Could you check a few things on this drawing? It's one solid part, dimensions in mm from its lowest x, y, z. Give positions to 0.01 mm unless a question says otherwise; leave off trailing zeros. Answer as a JSON object with one key per item and string values.
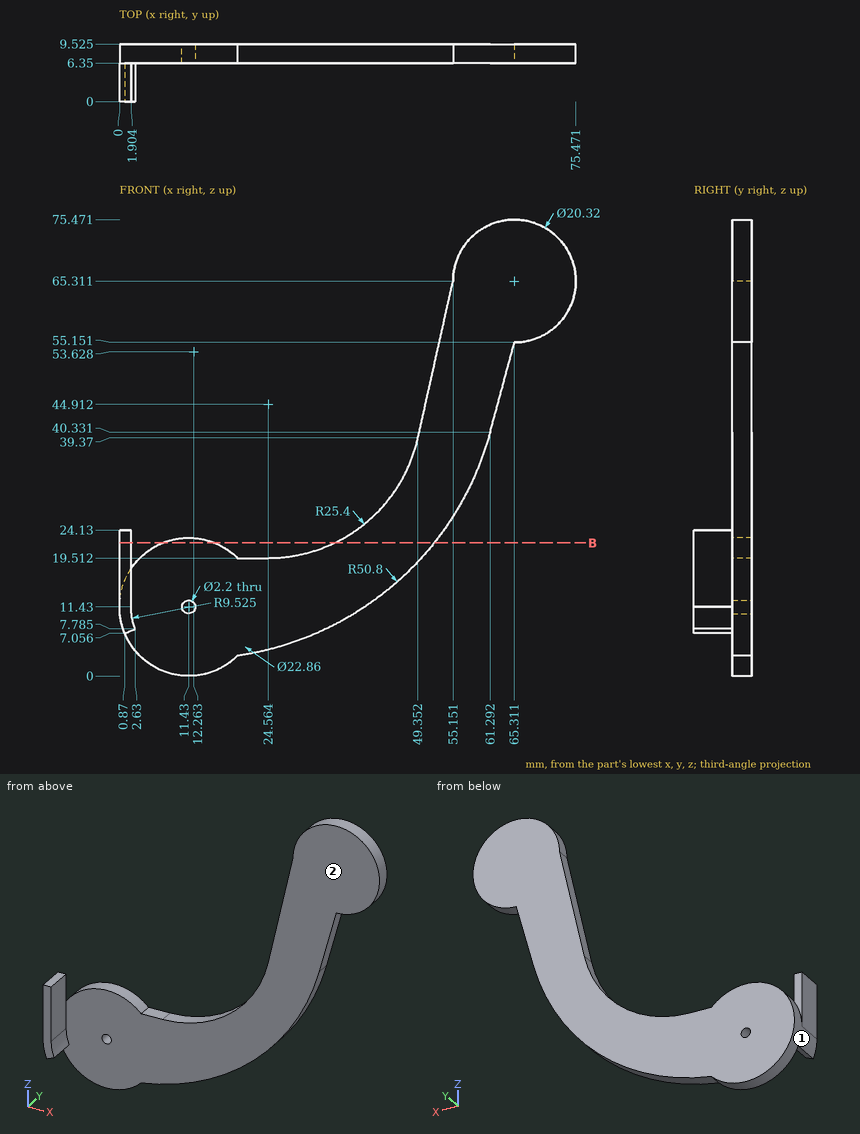
1. If we mould it in two halves opening along X, with no side actions, what happens to the marked faces 1 and 2? For each: +X half, -X half, draft (parallel to the pull), parting line (faces both ways), or undercut.
Worked answers:
{"face 1": "undercut", "face 2": "draft"}
2. Please list where these lines run through material, in increasing order: L1, parallel to Z at x = 11.43, y = 8.3; L2, parallel to X at y = 2.25, z = 22.5 (1 decimal); L3, parallel to Z at x = 10.5, y = 6.5 (1 decimal).
Worked answers:
{"L1": "0 to 10.33, 12.53 to 22.86", "L2": "0 to 1.9", "L3": "0 to 10.8, 12 to 22.8"}
3. Will these pins go through, and if not, where does the flat tip stop? pin 1 Ø1.5 at (y, z) = (5.5, 21.5) entering from +X; pin 2 Ø2 at (x, y) = (14.5, 6) entering from -Z; pin 3 Ø4 at (x, z) = (60.5, 39.5) entering from -Y.
Worked answers:
{"pin 1": "x = 1.9", "pin 2": "z = 0.2", "pin 3": "y = 6.35"}
4. If we section it at B-B on z = 22: Count the separate pieces of the cut face and the enclosed holes in it.
Worked answers:
{"separate pieces": "3", "enclosed holes": "0"}
